For this review, take the finished solid that the model builds, in its own axes (mm). A direction names the side the tool comes from. Round coordinates to 2 decimals unless told otherwise and drop trailing zeros. Write each loop counter-clockwise with the first axis right and the second up, starting at its lowest first coordinate (ties: lowest second). Pieces come first, ordered by that corner, then holes.
Autodesk Inventor part; units mm, degrees
ref_plane "YZ Plane" through (0, 0, 0) normal (1, 0, 0) x (0, 1, 0)
ref_plane "XZ Plane" through (0, 0, 0) normal (0, 1, 0) x (-1, 0, 0)
ref_plane "XY Plane" through (0, 0, 0) normal (0, 0, 1) x (1, 0, 0)
sketch "Sketch1" plane through (0, 0, 0) normal (0, 1, 0) x (-1, 0, 0)
  line L0 (4.808, 48.5926) -> (7.058, 47.7737)
  line L1 (4.808, 49.4815) -> (4.808, 48.5926)
  line L2 (4.808, 49.4815) -> (7.058, 50.2996)
  line L3 (7.058, 50.2996) -> (7.058, 50.9144)
  line L4 (4.808, 51.7333) -> (7.058, 50.9144)
  line L5 (4.808, 52.6222) -> (4.808, 51.7333)
  line L6 (4.808, 52.6222) -> (7.058, 53.4403)
  line L7 (7.058, 53.4403) -> (7.058, 54.0552)
  line L8 (4.808, 54.8741) -> (7.058, 54.0552)
  line L9 (4.808, 55.763) -> (4.808, 54.8741)
  line L10 (4.808, 55.763) -> (7.058, 56.581)
  line L11 (7.058, 56.581) -> (7.058, 57.1959)
  line L12 (4.808, 58.0148) -> (7.058, 57.1959)
  line L13 (4.808, 58.9037) -> (4.808, 58.0148)
  line L14 (4.808, 58.9037) -> (7.058, 59.7218)
  line L15 (7.058, 59.7218) -> (7.058, 60.3366)
  line L16 (4.808, 61.1556) -> (7.058, 60.3366)
  line L17 (4.808, 62.0444) -> (4.808, 61.1556)
  line L18 (4.808, 62.0444) -> (7.058, 62.8625)
  line L19 (7.058, 62.8625) -> (7.058, 63.4774)
  line L20 (4.808, 64.2963) -> (7.058, 63.4774)
  line L21 (4.808, 65.1852) -> (4.808, 64.2963)
  line L22 (4.808, 65.1852) -> (7.058, 66.0033)
  line L23 (7.058, 66.0033) -> (7.058, 66.6181)
  line L24 (4.808, 67.437) -> (7.058, 66.6181)
  line L25 (4.808, 68.3259) -> (4.808, 67.437)
  line L26 (4.808, 68.3259) -> (7.058, 69.144)
  line L27 (7.058, 69.144) -> (7.058, 69.7588)
  line L28 (4.808, 70.5778) -> (7.058, 69.7588)
  line L29 (4.808, 71.4667) -> (4.808, 70.5778)
  line L30 (4.808, 71.4667) -> (7.058, 72.2847)
  line L31 (7.058, 72.2847) -> (7.058, 72.8996)
  line L32 (4.808, 73.7185) -> (7.058, 72.8996)
  line L33 (4.808, 74.6074) -> (4.808, 73.7185)
  line L34 (4.808, 74.6074) -> (7.058, 75.4255)
  line L35 (7.058, 75.4255) -> (7.058, 76.0403)
  line L36 (4.808, 76.8593) -> (7.058, 76.0403)
  line L37 (4.808, 77.7481) -> (4.808, 76.8593)
  line L38 (4.808, 77.7481) -> (7.058, 78.5662)
  line L39 (7.058, 78.5662) -> (7.058, 79.1811)
  line L40 (4.808, 80) -> (7.058, 79.1811)
  line L41 (-3, 80) -> (4.808, 80)
  line L42 (-3, 80) -> (-3, -1.5)
  arc A0 (-3, -1.5) -> (-1, -3.5) centre (-1, -1.5) ccw
  line L43 (1, -3.5) -> (-1, -3.5)
  arc A1 (1, -3.5) -> (3, -1.5) centre (1, -1.5) ccw
  line L44 (3, 43.2) -> (3, -1.5)
  line L45 (4.808, 43.2) -> (7.058, 44.0181)
  line L46 (7.058, 44.0181) -> (7.058, 44.6329)
  line L47 (4.808, 45.4519) -> (7.058, 44.6329)
  line L48 (4.808, 46.3407) -> (4.808, 45.4519)
  line L49 (4.808, 46.3407) -> (7.058, 47.1588)
  line L50 (7.058, 47.1588) -> (7.058, 47.7737)
  circle A2 centre (0, 0) radius 1
  arc A3 (-0.392, 47.5) -> (2.308, 47.5) centre (0.958, 47.5) ccw
  line L51 (-0.392, 75.5) -> (-0.392, 47.5)
  arc A4 (2.308, 75.5) -> (-0.392, 75.5) centre (0.958, 75.5) ccw
  line L52 (2.308, 75.5) -> (2.308, 47.5)
  line L53 (3, 43.2) -> (4.808, 43.2)
  point P0 (4.808, 77.3037)
  point P1 (4.808, 49.037)
  point P2 (0.904, 80)
  dimension "d0" = 2.25
  dimension "d3" = 28
  dimension "d4" = 2.7
  dimension "d7" = 2.5
  dimension "d8" = 4.3
  dimension "d11" = 6
  dimension "d12" = 3
  dimension "d13" = 3.5
  dimension "d15" = 0.6149
  dimension "d16" = 0.8889
  dimension "d17" = 20
  dimension "d28" = 4.808
  dimension "d29" = 36.8
  dimension "d30" = 4.5
  dimension "d31" = 83.5
  dimension "d32" = 2
  dimension "d33" = 2
  dimension "d34" = 2
  dimension "d37" = 2.608
  dimension "d38" = 2
extrude "Extrusion1" add sketch "Sketch1" along normal blind 3
fillet "Fillet1" radius 2 1 edges at (3, 1.5, 80)
equation "\"dist_finEngrane_tornilloSujetadorPilot\" = 4.808"
properties part number "cremallera_v2"
(1) Mouldability with a two-part tool opening along Z and no side actions: class faces 6 (the face through (-2, 1, 80)), 7 (the face through (-4, 1, 43.2)), 8 (the face through (-5.917, 1.479, 76.456)), 9 (the face through (-5.92, 1.48, 68.73)) as pulls with the +Z half, pulls with the -Z half, needs draft (parallel to the pull), parting line crosses it, or undercut.
Geometry check:
face 6: pulls with the +Z half
face 7: pulls with the -Z half
face 8: undercut
face 9: undercut
(2) We need section A-A, the plane z = 0. Give the boundary of the cut face in (x, y).
Geometry check:
outline: (-3, 0) - (-1, 0) - (-1, 3) - (-3, 3) - close; (1, 0) - (3, 0) - (3, 3) - (1, 3) - close
(3) For pin 1 Ø1 at (x, z) = (-1, 70) entering from +Y; pin 2 Ø1.5 at (y, z) = (1.5, 25.5) entering from -X; pin 3 Ø0.9 at (x, y) = (-4.5, 1) entering from -Z; pin 4 Ø0.7 at (y, z) = (1.5, 71) entering from -X, all flat-tipped, find the tip position at first contact; note any pin that passes through.
Geometry check:
pin 1: passes through
pin 2: stops at x = -3
pin 3: stops at z = 43.2
pin 4: stops at x = -4.81
(4) We need section D-D, the plane z = 24. Give the boundary of the cut face in (x, y).
Geometry check:
outline: (-3, 0) - (3, 0) - (3, 3) - (-3, 3) - close
(5) We need section B-B, the plane y = 1.8. State how many separate pieces and enclosed holes the cut face has, and give its area (3 significant figures).
Geometry check:
separate pieces: 1
enclosed holes: 2
area: 519 mm2
(6) For line 1 along Z through (x, y) = (0, 0.85); line 2 along Z through (x, y) = (-0.5, 2.8); line 3 along X through (y, z) = (2.3, 74.5), list the stretches that pass through material, from the lowest coordinate up.
Geometry check:
line 1: z = -3.5 to -1, 1 to 46.55, 76.45 to 80
line 2: z = -3.5 to -0.87, 0.87 to 46.23, 76.77 to 80
line 3: x = -4.81 to -2.31, 0.39 to 3
(7) For faces 1 (the face through (-3, 1, 21)), 2 (the face through (-2.308, 1, 62)), 3 (the face through (-1, 3, 39)), 4 (the face through (2.4, 1.52, 79.43)), 5 (the face through (-5.917, 1.479, 70.174)), list the 3-axis set-ups (+Z, -Z, +X, -X, +Y, -Y) from which the entire face can be reached by the end or side of a thin tool; tool diameter is ignored.
Geometry check:
face 1: -Z, -X, +Y, -Y
face 2: +Y, -Y
face 3: +Z, -Z, +X, -X, +Y
face 4: +Z, +X, +Y, -Y
face 5: -X, +Y, -Y
